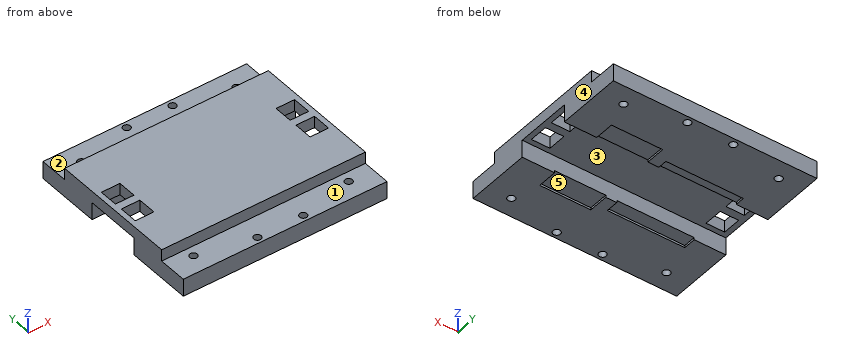
```python
from build123d import *

# Parameters (mm, degrees)
F0_W      = 139.446
F0_H      = 20
F1_DEPTH  = 63.5
F2_W      = 139.446
F2_H      = 19.567398
F3_DEPTH  = 8.000009
F5_W      = 12.7
F5_H      = 12.7
F6_DEPTH  = 21.844
F8_R      = 2.54
F9_DEPTH  = 76.2
F13_W     = 53
F13_H     = 53
F13_W_2   = 35
F13_H_2   = 65
F14_DEPTH = 1.5
F15_DEPTH = 12.000001


with BuildPart() as f1:
    # F0 (on Front) → F1 (new body, symmetric)
    with BuildSketch(Plane.XZ):
        Rectangle(F0_W, F0_H)
    extrude(amount=F1_DEPTH, both=True)

    # F2 (on face) → F3 (cut)
    with BuildSketch(Plane.XY.offset(10)):
        with Locations((0, -53.716301)):
            Rectangle(F2_W, F2_H)
    extrude(amount=-F3_DEPTH, mode=Mode.SUBTRACT)

    # F4: F1 across plane


with BuildPart() as f1_1:
    add(f1.part)
    add(f1.part.mirror(Plane.XZ), mode=Mode.INTERSECT)

    # F5 (on face) → F6 (cut)
    with BuildSketch(Plane.XY.offset(10)):
        with Locations((59.793662, -9.017324)):
            Rectangle(F5_W, F5_H)
    extrude(amount=-F6_DEPTH, mode=Mode.SUBTRACT)

    # F8 (on face) → F9 (cut)
    with BuildSketch(Plane.XY.offset(1.999991)):
        with Locations((53.08092, -50.8)):
            Circle(F8_R)
        with Locations((15.705684, -59.173669)):
            Circle(F8_R)
    extrude(amount=-F9_DEPTH, mode=Mode.SUBTRACT)

    # F10: F1 across plane


with BuildPart() as f1_2:
    add(f1_1.part)
    add(f1_1.part.mirror(Plane.XZ), mode=Mode.INTERSECT)

    # F11: F1 across plane


with BuildPart() as f1_3:
    add(f1_2.part)
    add(f1_2.part.mirror(Plane.YZ), mode=Mode.INTERSECT)

    # F13 (on face) → F14 (cut)
    with BuildSketch(Plane(origin=(0, 0, -10), x_dir=(1, 0, 0), z_dir=(0, 0, -1))):
        with Locations((-21.51399, 1)):
            Rectangle(F13_W, F13_H)
        with Locations((29.994886, 0)):
            Rectangle(F13_W_2, F13_H_2)
    extrude(amount=-F14_DEPTH, mode=Mode.SUBTRACT)

    # F12 (on face) → F15 (cut)
    with BuildSketch(Plane(origin=(0, 0, -10), x_dir=(1, 0, 0), z_dir=(0, 0, -1))):
        Polygon((69.723, -19.123085), (69.723, 18.976915), (1.722882, 18.976915), (-69.723, 18.976915), (-69.723, -19.123085), (1.722882, -19.123085), align=None)
    extrude(amount=-F15_DEPTH, mode=Mode.SUBTRACT)


solid = f1_3.part
```
Source: CAD feature listing. Evaluate the final solid. Frame: model axes, mm. Face numbers are marked on the shaded views. A direction names the side the tool comes from. Coordinates: 2 decimals unless noted, no trailing zeros. Write each loop counter-clockwise with the first axis right and the second up, starting at its lowest first coordinate (ties: lowest second). Pieces come first, ordered by that corner, then holes. Notation, with made-up numbers: (8.25, 86) - (52.25, 86) arc R35 ccw to (52.25, 125) - close; hole circle Ø8 at (66, 38.5). An arc over 180 degrees is marked (long way). Answer as a JSON object with one key per item and string values.
Q1. Section query B-B, the plane z = -2.25. State how many separate pieces and enclosed holes the cut face has, plus the area to 3 significant figures.
Ans:
{"separate pieces": "2", "enclosed holes": "8", "area": "12,200 mm2"}
Q2. Material intervals for line 1 (Y direction, x = 56.5, z = 8.5); line 2 (X direction, y = 50.8, z = -3.25); line 3 (Y direction, x = 4, z = -3), sorted ascending. Write a range as [from, to].
Ans:
{"line 1": "y = [-43.93, -15.37], [-2.67, 2.67], [15.37, 43.93]", "line 2": "x = [-69.72, -55.62], [-50.54, 50.54], [55.62, 69.72]", "line 3": "y = [-63.5, -18.98], [19.12, 63.5]"}
Q3. Section query A-A, the plane y = 50.8. Output: boundary loops of the cut face in (x, z).
Ans:
{"outline": "(-69.72, -10) - (-55.62, -10) - (-55.62, 2) - (-69.72, 2) - close; (-50.54, -10) - (50.54, -10) - (50.54, 2) - (-50.54, 2) - close; (55.62, -10) - (69.72, -10) - (69.72, 2) - (55.62, 2) - close"}
Q4. Section query D-D, the plane y = 5. Output: boundary loops of the cut face in (x, z).
Ans:
{"outline": "(-69.72, 2) - (-66.14, 2) - (-66.14, 10) - (-69.72, 10) - close; (-53.44, 2) - (53.44, 2) - (53.44, 10) - (-53.44, 10) - close; (66.14, 2) - (69.72, 2) - (69.72, 10) - (66.14, 10) - close"}
Q5. Section query C-C, the plane x = 59.5. Output: boundary loops of the cut face in (y, z), plus the area to 3 significant figures.
Ans:
{"outline": "(-63.5, -10) - (-18.98, -10) - (-18.98, 2) - (-15.37, 2) - (-15.37, 10) - (-43.93, 10) - (-43.93, 2) - (-63.5, 2) - close; (-2.67, 2) - (2.67, 2) - (2.67, 10) - (-2.67, 10) - close; (15.37, 2) - (19.12, 2) - (19.12, -10) - (63.5, -10) - (63.5, 2) - (43.93, 2) - (43.93, 10) - (15.37, 10) - close", "area": "1,570 mm2"}
Q6. Draft query along Y for the marked faces 4 and 5. Return one class per face: released by +Y, released by -Y, zero draft, split by the parting line, or undercut.
Ans:
{"face 4": "zero draft", "face 5": "undercut"}
Q7. Set-up query: the marked faces 1, 2 and 3. Return all of +Z, -Z, +X, -X, +Y, -Y with unobstructed straight access to the full face (end or side cutting, diameter ignored); none if empty.
Ans:
{"face 1": "+Z, +X, -X, -Y", "face 2": "+Z, +X, -X, +Y", "face 3": "-Z, +X, -X"}
Q8. First-contact query: pin 1 Ø6.5 at (x, y) = (33.5, 25) entering from -Z; pin 2 Ø6 at (x, y) = (15.71, -59.17) entering from +Z; pin 3 Ø9 at (x, z) = (-58, 4.5) entering from -Y; pin 4 Ø4 at (x, z) = (-59.5, 7) entering from +Y. Flat tips, straight axial feed; report the tip coordinate or a pass-through.
Ans:
{"pin 1": "stops at z = -8.5", "pin 2": "stops at z = 2", "pin 3": "stops at y = -63.5", "pin 4": "stops at y = 43.93"}
